Source: CAD feature listing. Evaluate the final solid. Frame: model axes, mm. A direction names the side the tool comes from. Coordinates: 2 decimals unless noted, no trailing zeros. Loops run counter-clockwise (first coordinate to the right, second up) from the corner with the lowest first, then second, coordinate; pieces in that order, holes last.
Item 1: Section query D-D, the plane z = -34.5. Return the cut outline in (x, y).
Item 2: Reachability of faces 1 (the flat face through (63, 0, -29)), 2 (the flat face through (39, 22.4, -2)), 3 (the flat face through (63, -1, -50.8)), 4 (the cylindrical face through (73.113, 12.947, -1.521)), 5 (the cylindrical face through (12.46, -1.52, -38.65)) from +Z, -Z, +X, -X, +Y, -Y: full face, straight path, thin tool, end or side. Return the list, or none.
Item 3: Pull-direction query (X, two-part tool) for faces 6 (the flat face through (0, -1, -16)), 7 (the flat face through (127, -0.3, -14.2)), 8 (the flat face through (102, 47.8, -2)), 9 (the cylindrical face through (87.777, 21.825, -1.521)); classes: +X half, -X half, draft (parallel to the pull), parting line (faces both ways), or undercut.
Item 4: Section query B-B, the plane y = 28.75. Return the cut outline in (x, z).
Item 5: Line query: probe 1 along Z at (x, y) = (50.5, 7); probe 2 along Z at (x, y) = (35.5, -0.5). Output: solid intervals per line, ascending.
Item 6: Section query C-C, the plane x = 101.6. Return the cut outline in (y, z), then the cut area to 3 significant figures.
Item 7: Pin query (flat end, axial travel): pin 1 Ø12 at (x, z) = (40, -19.5) entering from +Y; pin 2 Ø2.5 at (x, z) = (26.5, -1) entering from +Y; pin 3 Ø2.5 at (y, z) = (41, -2) entering from -X. Return the tip coordinate at first contact, or that it passes through.
Item 8: Section query A-A, the plane x = 51.5. Return the cut outline in (y, z), then the cut area to 3 significant figures.
```python
from build123d import *

# Parameters (mm, degrees)
SKETCH1_W                    = 127
SKETCH1_H                    = 50.8
BASE_FLANGE1_DEPTH           = 3
EDGE_FLANGE1_STRIP_W         = 18
EDGE_FLANGE1_STRIP_H         = 3
EDGE_FLANGE1_STRIP_CUT_DEPTH = 127
EDGE_FLANGE1_DEPTH           = 127
UNFOLD1_DEPTH                = 127
UNFOLD1_2_DEPTH              = 127
SKETCH9_R                    = 11.25
SKETCH9_W                    = 76.2
SKETCH9_H                    = 25.4
CUT_EXTRUDE1_DEPTH           = 137.816080926
M3_CLEARANCE_HOLE1_D         = 3.4
M3_CLEARANCE_HOLE1_DEPTH     = 7.62
M3_CLEARANCE_HOLE1_TIP       = 1.021463052
M3_CLEARANCE_HOLE2_D         = 3.4
M3_CLEARANCE_HOLE2_DEPTH     = 7.62
M3_CLEARANCE_HOLE2_TIP       = 1.021463052
FOLD1_START                  = -0.61644
FOLD1_OUTLINE_W              = 127
FOLD1_OUTLINE_H              = 3
FOLD1_DEPTH                  = 46.485023471
FOLD1_START_2                = -3
FOLD1_2_OUTLINE_R            = 1.7
FOLD1_2_OUTLINE_R_2          = 11.25
FOLD1_2_DEPTH                = 0.01644
FOLD1_START_3                = -6
FOLD1_3_OUTLINE_R            = 1.7
FOLD1_3_OUTLINE_R_2          = 11.25
FOLD1_3_DEPTH                = 6
FOLD1_4_DEPTH                = 127


with BuildPart() as part:
    # Base-Flange1: sheet metal written as solids
    # Sketch1 → Base-Flange1 (new body)
    with BuildSketch(Plane(origin=(0, 0, 0), x_dir=(1, 0, 0), z_dir=(0, 1, 0))):
        with Locations((63.5, 25.4)):
            Rectangle(SKETCH1_W, SKETCH1_H)
    extrude(amount=-BASE_FLANGE1_DEPTH)

    # Edge-Flange1: sheet metal written as solids
    # Edge-Flange1 strip (on a plane across the edge) → Edge-Flange1 strip cut (cut)
    with BuildSketch(Plane(origin=(0, 0, 0), x_dir=(0, 0, -1), z_dir=(1, 0, 0))):
        with Locations((-3, -1.5)):
            Rectangle(EDGE_FLANGE1_STRIP_W, EDGE_FLANGE1_STRIP_H)
    extrude(amount=EDGE_FLANGE1_STRIP_CUT_DEPTH, mode=Mode.SUBTRACT)

    # Edge-Flange1 section (on a plane across the edge) → Edge-Flange1 (add)
    with BuildSketch(Plane(origin=(0, 0, 0), x_dir=(0, 0, -1), z_dir=(1, 0, 0))):
        with BuildLine():
            Line((0, 3), (0, 47.8))
            Line((0, 47.8), (3, 47.8))
            Line((3, 47.8), (3, 3))
            ThreePointArc((3, 3), (3.878679656, 0.878679656), (6, 0))
            Line((6, 0), (6, -3))
            ThreePointArc((6, -3), (1.757359313, -1.242640687), (0, 3))
        make_face()
    extrude(amount=EDGE_FLANGE1_DEPTH)

    # Unfold1: read off the stored shape, not the designer's step
    # Unfold1 outline → Unfold1 (cut)
    with BuildSketch(Plane.YZ):
        with BuildLine():
            ThreePointArc((3, 0), (1.447085729, -0.204445042), (0, -0.803847577))
            Line((0, -0.803847577), (0, -6))
            ThreePointArc((0, -6), (0.878679656, -3.878679656), (3, -3))
            Line((3, -3), (47.8, -3))
            Line((47.8, -3), (47.8, 0))
            Line((47.8, 0), (3, 0))
        make_face()
    extrude(amount=UNFOLD1_DEPTH, mode=Mode.SUBTRACT)

    # Unfold1 2 outline → Unfold1 2 (add)
    with BuildSketch(Plane.YZ):
        with BuildLine():
            Line((-3, 45.868583471), (-3, -6))
            ThreePointArc((-3, -6), (-2.196152423, -3), (0, -0.803847577))
            Line((0, -0.803847577), (0, 45.868583471))
            Line((0, 45.868583471), (-3, 45.868583471))
        make_face()
    extrude(amount=UNFOLD1_2_DEPTH)

    # Sketch9 → Cut-Extrude1 (cut, through all)
    with BuildSketch(Plane(origin=(0, 0, 0), x_dir=(1, 0, 0), z_dir=(0, 1, 0))):
        with Locations(Location((101.6, -26.818583471, 0), (0, 0, 270))):
            Circle(SKETCH9_R)
        with Locations((38.1, -33.168583471)):
            Rectangle(SKETCH9_W, SKETCH9_H)
        with BuildLine():
            Line((6.35, -7.679683471), (69.85, -7.679683471))
            ThreePointArc((69.85, -7.679683471), (73.1139, -10.943583471), (69.85, -14.207483471))
            Line((69.85, -14.207483471), (6.35, -14.207483471))
            ThreePointArc((6.35, -14.207483471), (3.0861, -10.943583471), (6.35, -7.679683471))
        make_face()
    extrude(amount=-CUT_EXTRUDE1_DEPTH, mode=Mode.SUBTRACT)

    # M3 Clearance Hole1
    with Locations(Plane(origin=(0, 0, 0), x_dir=(1, 0, 0), z_dir=(0, 1, 0))):
        with Locations((109.1, -13.828202414), (101.6, -40.818583471), (109.1, -39.808964527), (89.475644347, -19.818583471), (86.6, -26.818583471), (113.724355653, -19.818583471)):
            Hole(M3_CLEARANCE_HOLE1_D / 2, depth=M3_CLEARANCE_HOLE1_DEPTH)
            with Locations((0, 0, -(M3_CLEARANCE_HOLE1_DEPTH + M3_CLEARANCE_HOLE1_TIP / 2))):  # 118° drill point
                Cone(0, M3_CLEARANCE_HOLE1_D / 2, M3_CLEARANCE_HOLE1_TIP, mode=Mode.SUBTRACT)

    # M3 Clearance Hole2
    with Locations(Plane(origin=(0, 0, 0), x_dir=(1, 0, 0), z_dir=(0, 1, 0))):
        with Locations((11.1125, 39.6875), (115.8875, 39.6875), (115.8875, 11.1125), (11.1125, 11.1125)):
            Hole(M3_CLEARANCE_HOLE2_D / 2, depth=M3_CLEARANCE_HOLE2_DEPTH)
            with Locations((0, 0, -(M3_CLEARANCE_HOLE2_DEPTH + M3_CLEARANCE_HOLE2_TIP / 2))):  # 118° drill point
                Cone(0, M3_CLEARANCE_HOLE2_D / 2, M3_CLEARANCE_HOLE2_TIP, mode=Mode.SUBTRACT)

    # Fold1: read off the stored shape, not the designer's step
    # Fold1 outline → Fold1 (cut)
    with BuildSketch(Plane.XY.offset(FOLD1_START)):
        with Locations((63.5, -1.5)):
            Rectangle(FOLD1_OUTLINE_W, FOLD1_OUTLINE_H)
    extrude(amount=FOLD1_DEPTH, mode=Mode.SUBTRACT)

    # Fold1 2 outline → Fold1 2 (add)
    with BuildSketch(Plane.XY.offset(FOLD1_START_2)):
        Polygon((0, 22.4), (0, 0), (127, 0), (127, 47.8), (76.2, 47.8), (76.2, 22.4), align=None)
        with BuildLine():
            Line((69.85, 9.6111), (6.35, 9.6111))
            ThreePointArc((6.35, 9.6111), (3.0861, 12.875), (6.35, 16.1389))
            Line((6.35, 16.1389), (69.85, 16.1389))
            ThreePointArc((69.85, 16.1389), (73.1139, 12.875), (69.85, 9.6111))
        make_face(mode=Mode.SUBTRACT)
        with Locations((89.475644347, 21.75)):
            Circle(FOLD1_2_OUTLINE_R, mode=Mode.SUBTRACT)
        with Locations((109.1, 15.759618943)):
            Circle(FOLD1_2_OUTLINE_R, mode=Mode.SUBTRACT)
        with Locations((113.724355653, 21.75)):
            Circle(FOLD1_2_OUTLINE_R, mode=Mode.SUBTRACT)
        with Locations((86.6, 28.75)):
            Circle(FOLD1_2_OUTLINE_R, mode=Mode.SUBTRACT)
        with Locations((101.6, 28.75)):
            Circle(FOLD1_2_OUTLINE_R_2, mode=Mode.SUBTRACT)
        with Locations((101.6, 42.75)):
            Circle(FOLD1_2_OUTLINE_R, mode=Mode.SUBTRACT)
        with Locations((109.1, 41.740381057)):
            Circle(FOLD1_2_OUTLINE_R, mode=Mode.SUBTRACT)
    extrude(amount=FOLD1_2_DEPTH)

    # Fold1 3 outline → Fold1 3 (add)
    with BuildSketch(Plane.XY.offset(FOLD1_START_3)):
        Polygon((0, 22.4), (0, 0), (127, 0), (127, 47.8), (76.2, 47.8), (76.2, 22.4), align=None)
        with BuildLine():
            Line((69.85, 9.6111), (6.35, 9.6111))
            ThreePointArc((6.35, 9.6111), (3.0861, 12.875), (6.35, 16.1389))
            Line((6.35, 16.1389), (69.85, 16.1389))
            ThreePointArc((69.85, 16.1389), (73.1139, 12.875), (69.85, 9.6111))
        make_face(mode=Mode.SUBTRACT)
        with Locations((89.475644347, 21.75)):
            Circle(FOLD1_3_OUTLINE_R, mode=Mode.SUBTRACT)
        with Locations((109.1, 15.759618943)):
            Circle(FOLD1_3_OUTLINE_R, mode=Mode.SUBTRACT)
        with Locations((113.724355653, 21.75)):
            Circle(FOLD1_3_OUTLINE_R, mode=Mode.SUBTRACT)
        with Locations((86.6, 28.75)):
            Circle(FOLD1_3_OUTLINE_R, mode=Mode.SUBTRACT)
        with Locations((101.6, 28.75)):
            Circle(FOLD1_3_OUTLINE_R_2, mode=Mode.SUBTRACT)
        with Locations((101.6, 42.75)):
            Circle(FOLD1_3_OUTLINE_R, mode=Mode.SUBTRACT)
        with Locations((109.1, 41.740381057)):
            Circle(FOLD1_3_OUTLINE_R, mode=Mode.SUBTRACT)
    extrude(amount=FOLD1_3_DEPTH)

    # Fold1 4 outline → Fold1 4 (cut)
    with BuildSketch(Plane.YZ):
        with BuildLine():
            ThreePointArc((-3, -6), (-1.242640687, -1.757359313), (3, 0))
            Line((3, 0), (0, 0))
            Line((0, 0), (0, -0.61644))
            Line((0, -0.61644), (-3, -0.61644))
            Line((-3, -0.61644), (-3, -6))
        make_face()
        with BuildLine():
            ThreePointArc((3, -3), (0.878679656, -3.878679656), (0, -6))
            Line((0, -6), (47.8, -6))
            Line((47.8, -6), (47.8, -3))
            Line((47.8, -3), (3, -3))
        make_face()
    extrude(amount=FOLD1_4_DEPTH, mode=Mode.SUBTRACT)


solid = part.part
```
Verdict:
1. outline: (0, -3) - (127, -3) - (127, 0) - (0, 0) - close
2. face 1: -Z, +X, -X, +Y
2. face 2: +Z, -Z, -X, +Y
2. face 3: -Z, +X, -X, +Y, -Y
2. face 4: +Z, -Z
2. face 5: +Y, -Y
3. face 6: -X half
3. face 7: +X half
3. face 8: draft
3. face 9: undercut
4. outline: (76.2, -3) - (84.9, -3) - (84.9, 0) - (76.2, 0) - close; (88.3, -3) - (90.35, -3) - (90.35, 0) - (88.3, 0) - close; (112.85, -3) - (127, -3) - (127, 0) - (112.85, 0) - close
5. probe 1: z = -3 to 0
5. probe 2: z = -50.8 to -1.13
6. outline: (-3, -50.8) - (0, -50.8) - (0, -6) arc R3 cw to (3, -3) - (17.5, -3) - (17.5, 0) - (3, 0) arc R6 ccw to (-3, -6) - close; (40, -3) - (41.05, -3) - (41.05, 0) - (40, 0) - close; (44.45, -3) - (47.8, -3) - (47.8, 0) - (44.45, 0) - close
6. area: 212 mm2
7. pin 1: stops at y = 0
7. pin 2: stops at y = 22.4
7. pin 3: stops at x = 76.2
8. outline: (-3, -50.8) - (0, -50.8) - (0, -6) arc R3 cw to (3, -3) - (9.61, -3) - (9.61, 0) - (3, 0) arc R6 ccw to (-3, -6) - close; (16.14, -3) - (22.4, -3) - (22.4, 0) - (16.14, 0) - close
8. area: 194 mm2
